```python
from build123d import *

# Parameters (mm, degrees)
SKETCH_1_W          = 87
SKETCH_1_H          = 63
SKETCH_1_W_2        = 83
SKETCH_1_H_2        = 59
EXTRUDE_1_DEPTH     = 5
SKETCH_2_W          = 87
SKETCH_2_H          = 63
EXTRUDE_2_DEPTH     = 2
SKETCH_3_W          = 2.764626384
SKETCH_3_H          = 4.6515936
CUT_EXTRUDE_1_DEPTH = 2
FILLET_1_R          = 2
SKETCH_4_W          = 27.388964673
SKETCH_4_H          = 3.905856672
SKETCH_4_W_2        = 13.70635998
SKETCH_4_H_2        = 4.505719406
SKETCH_4_W_3        = 11.157018238
SKETCH_4_H_3        = 2.851387493
SKETCH_4_W_4        = 3.109085913
SKETCH_4_H_4        = 44.489819457
EXTRUDE_3_DEPTH     = 3.3
SKETCH_5_R          = 2.75
CUT_EXTRUDE_2_DEPTH = 10


with BuildPart() as part:
    # 草图1 → 凸台-拉伸1 (new body)
    with BuildSketch(Plane(origin=(0, 0, 0), x_dir=(0, 0, -1), z_dir=(1, 0, 0))):
        with Locations((3.90387463, 17.013155975)):
            Rectangle(SKETCH_1_W, SKETCH_1_H)
        with Locations((3.90387463, 17.013155975)):
            Rectangle(SKETCH_1_W_2, SKETCH_1_H_2, mode=Mode.SUBTRACT)
    extrude(amount=EXTRUDE_1_DEPTH)

    # 草图2 → 凸台-拉伸2 (add)
    with BuildSketch(Plane(origin=(5, 0, 0), x_dir=(0, 0, -1), z_dir=(1, 0, 0))):
        with Locations((3.90387463, 17.013155975)):
            Rectangle(SKETCH_2_W, SKETCH_2_H)
    extrude(amount=EXTRUDE_2_DEPTH)

    # 草图3 → 切除-拉伸1 (cut)
    with BuildSketch(Plane(origin=(0, 0, -47.40387463), x_dir=(-1, 0, 0), z_dir=(0, 0, -1))):
        with Locations((-3.662779601, -6.806448474)):
            Rectangle(SKETCH_3_W, SKETCH_3_H)
    extrude(amount=-CUT_EXTRUDE_1_DEPTH, mode=Mode.SUBTRACT)

    # 圆角1
    # the kernel refuses this fillet: 2 mm, written as the material it takes off along each edge
    with BuildSketch(Plane(origin=(5, 46.513155975, -45.40387463), x_dir=(1, 0, 0), z_dir=(0, 1, 0))) as fillet_1_piece_1_section:
        Polygon((0, 0), (FILLET_1_R, 0), (FILLET_1_R, FILLET_1_R), (0, FILLET_1_R), align=None)
    fillet_1_piece_1 = extrude(amount=FILLET_1_R, mode=Mode.PRIVATE)
    fillet_1_piece_1 = fillet_1_piece_1 - Plane(origin=(5, 46.513155975, -45.40387463), x_dir=(-0.7071067811865475, 0, 0.7071067811865475), z_dir=(0, 1, 0)) * Sphere(FILLET_1_R, mode=Mode.PRIVATE)
    add(fillet_1_piece_1, mode=Mode.SUBTRACT)
    with BuildSketch(Plane(origin=(5, -12.486844025, -45.40387463), x_dir=(0, 0, -1), z_dir=(1, 0, 0))) as fillet_1_piece_2_section:
        Polygon((0, 0), (FILLET_1_R, 0), (FILLET_1_R, -FILLET_1_R), (0, -FILLET_1_R), align=None)
    fillet_1_piece_2 = extrude(amount=FILLET_1_R, mode=Mode.PRIVATE)
    fillet_1_piece_2 = fillet_1_piece_2 - Plane(origin=(5, -12.486844025, -45.40387463), x_dir=(0, 0.7071067811865474, 0.7071067811865476), z_dir=(1, 0, 0)) * Sphere(FILLET_1_R, mode=Mode.PRIVATE)
    add(fillet_1_piece_2, mode=Mode.SUBTRACT)
    with BuildSketch(Plane(origin=(5, -12.486844025, 37.59612537), x_dir=(1, 0, 0), z_dir=(0, 0, 1))) as fillet_1_piece_3_section:
        Polygon((0, 0), (FILLET_1_R, 0), (FILLET_1_R, -FILLET_1_R), (0, -FILLET_1_R), align=None)
    fillet_1_piece_3 = extrude(amount=FILLET_1_R, mode=Mode.PRIVATE)
    fillet_1_piece_3 = fillet_1_piece_3 - Plane(origin=(5, -12.486844025, 37.59612537), x_dir=(-0.7071067811865475, 0.7071067811865475, 0), z_dir=(0, 0, 1)) * Sphere(FILLET_1_R, mode=Mode.PRIVATE)
    add(fillet_1_piece_3, mode=Mode.SUBTRACT)
    with BuildSketch(Plane(origin=(5, 46.513155975, 37.59612537), x_dir=(0, 0, 1), z_dir=(0, 1, 0))) as fillet_1_piece_4_section:
        Polygon((0, 0), (FILLET_1_R, 0), (FILLET_1_R, FILLET_1_R), (0, FILLET_1_R), align=None)
    fillet_1_piece_4 = extrude(amount=FILLET_1_R, mode=Mode.PRIVATE)
    fillet_1_piece_4 = fillet_1_piece_4 - Plane(origin=(5, 46.513155975, 37.59612537), x_dir=(-0.7071067811865475, 0, -0.7071067811865475), z_dir=(0, 1, 0)) * Sphere(FILLET_1_R, mode=Mode.PRIVATE)
    add(fillet_1_piece_4, mode=Mode.SUBTRACT)
    with BuildSketch(Plane(origin=(5, 48.513155975, -47.40387463), x_dir=(0, 0, 1), z_dir=(-1, 0, 0)), Plane(origin=(5, -14.486844025, -47.40387463), x_dir=(0, 1, 0), z_dir=(-1, 0, 0)), Plane(origin=(-5, -14.486844025, 39.59612537), x_dir=(0, 1, 0), z_dir=(1, 0, 0)), Plane(origin=(-5, 48.513155975, 39.59612537), x_dir=(0, 0, -1), z_dir=(1, 0, 0))) as fillet_1_piece_5:
        with BuildLine():
            CenterArc((FILLET_1_R, -FILLET_1_R), FILLET_1_R, 90, 90)
            Line((0, -FILLET_1_R), (0, 0))
            Line((0, 0), (FILLET_1_R, 0))
        make_face()
    extrude(amount=10, mode=Mode.SUBTRACT)
    with BuildSketch(Plane(origin=(7, 48.513155975, 37.59612537), x_dir=(-1, 0, 0), z_dir=(0, 0, -1))) as fillet_1_piece_6:
        with BuildLine():
            CenterArc((FILLET_1_R, -FILLET_1_R), FILLET_1_R, 90, 90)
            Line((0, -FILLET_1_R), (0, 0))
            Line((0, 0), (FILLET_1_R, 0))
        make_face()
    extrude(amount=83, mode=Mode.SUBTRACT)
    with BuildSketch(Plane(origin=(7, 46.513155975, -47.40387463), x_dir=(0, 0, 1), z_dir=(0, -1, 0))) as fillet_1_piece_7:
        with BuildLine():
            CenterArc((FILLET_1_R, FILLET_1_R), FILLET_1_R, 180, 90)
            Line((0, FILLET_1_R), (0, 0))
            Line((0, 0), (FILLET_1_R, 0))
        make_face()
    extrude(amount=59, mode=Mode.SUBTRACT)
    with BuildSketch(Plane(origin=(7, -14.486844025, -45.40387463), x_dir=(0, 1, 0), z_dir=(0, 0, 1))) as fillet_1_piece_8:
        with BuildLine():
            CenterArc((FILLET_1_R, FILLET_1_R), FILLET_1_R, 180, 90)
            Line((0, FILLET_1_R), (0, 0))
            Line((0, 0), (FILLET_1_R, 0))
        make_face()
    extrude(amount=83, mode=Mode.SUBTRACT)
    with BuildSketch(Plane(origin=(7, -12.486844025, 39.59612537), x_dir=(-1, 0, 0), z_dir=(0, 1, 0))) as fillet_1_piece_9:
        with BuildLine():
            CenterArc((FILLET_1_R, -FILLET_1_R), FILLET_1_R, 90, 90)
            Line((0, -FILLET_1_R), (0, 0))
            Line((0, 0), (FILLET_1_R, 0))
        make_face()
    extrude(amount=59, mode=Mode.SUBTRACT)

    # 草图4 → 凸台-拉伸3 (add)
    with BuildSketch(Plane.ZY.offset(-5)):
        with Locations((13.694482337, -10.533915689)):
            Rectangle(SKETCH_4_W, SKETCH_4_H)
        with Locations((-38.55069464, 44.260296272)):
            Rectangle(SKETCH_4_W_2, SKETCH_4_H_2)
        with Locations((32.017616251, 45.087462229)):
            Rectangle(SKETCH_4_W_3, SKETCH_4_H_3)
        with Locations((36.041582414, 16.563258925)):
            Rectangle(SKETCH_4_W_4, SKETCH_4_H_4)
    extrude(amount=EXTRUDE_3_DEPTH)

    # 草图5 → 切除-拉伸2 (cut)
    with BuildSketch(Plane.ZY.offset(-5)):
        with Locations((-34.13110136, 33.698944985)):
            Circle(SKETCH_5_R)
        with Locations((26.3233521, 33.698944985)):
            Circle(SKETCH_5_R)
        with Locations((-34.13110136, 0.327366965)):
            Circle(SKETCH_5_R)
        with Locations((26.3233521, 0.327366965)):
            Circle(SKETCH_5_R)
    extrude(amount=-CUT_EXTRUDE_2_DEPTH, mode=Mode.SUBTRACT)


solid = part.part
```
Could you check a few things on this model? Use its own coordinates, in mm. A direction names the side the tool comes from. Give positions to 0.01 mm unless a question says otherwise; leave off trailing zeros. Loops run counter-clockwise (first coordinate to the right, second up) from the corner with the lowest first, then second, coordinate; pieces in that order, holes last. Notation, with made-up numbers: (27.5, 79) -> (32.5, 79) arc R13 cw to (32.5, 100) -> close; hole circle Ø4 at (77.5, 88.5). An arc over 180 degrees is marked (long way). Put each result on its own line as item: value.
(1) Imagine slicing it at B-B on z = -40.5. Write out the boundary of the cut face in (x, y), plus the area to 3 significant figures.
Computed:
outline: (0, -14.49) -> (5, -14.49) arc R2 ccw to (7, -12.49) -> (7, 46.51) arc R2 ccw to (5, 48.51) -> (0, 48.51) -> (0, 46.51) -> (1.7, 46.51) -> (1.7, 42.01) -> (5, 42.01) -> (5, -12.49) -> (0, -12.49) -> close
area: 159 mm^2
(2) Imagine slicing it at A-A on x = 4. Write out the boundary of the cut face in (y, z).
Computed:
outline: (-14.49, -45.4) arc R2 ccw to (-12.49, -47.4) -> (-9.13, -47.4) -> (-9.13, -45.4) -> (-12.49, -45.4) -> (-12.49, 0) -> (-8.58, 0) -> (-8.58, 27.39) -> (-12.49, 27.39) -> (-12.49, 37.6) -> (-5.68, 37.6) -> (-5.68, 34.49) -> (38.81, 34.49) -> (38.81, 37.6) -> (43.66, 37.6) -> (43.66, 26.44) -> (46.51, 26.44) -> (46.51, -31.7) -> (42.01, -31.7) -> (42.01, -45.4) -> (-4.48, -45.4) -> (-4.48, -47.4) -> (46.51, -47.4) arc R2 ccw to (48.51, -45.4) -> (48.51, 37.6) arc R2 ccw to (46.51, 39.6) -> (-12.49, 39.6) arc R2 ccw to (-14.49, 37.6) -> close
(3) Thinking about a two-plate mould opening in Y: for faces 1 (the face through (6.399, 16.6, 39.026)), 2 (the face through (2.535, 47.943, -46.802)), 3 (the face through (3, -8.581, 14)), 4 (the face through (4, -9.132, -46)), which applies, pulls with the +Y half, pulls with the -Y half, needs draft (parallel to the pull), parting line crosses it, or undercut?
Computed:
face 1: needs draft
face 2: pulls with the +Y half
face 3: undercut
face 4: undercut
(4) Imagine slicing it at C-C on y = 45.5. Write out the boundary of the cut face in (x, z), plus the area to 3 significant figures.
Computed:
outline: (0, -47.4) -> (5, -47.4) arc R2 ccw to (7, -45.4) -> (7, 37.6) arc R2 ccw to (5, 39.6) -> (0, 39.6) -> (0, 37.6) -> (1.7, 37.6) -> (1.7, 26.44) -> (5, 26.44) -> (5, -31.7) -> (1.7, -31.7) -> (1.7, -45.4) -> (0, -45.4) -> close
area: 274 mm^2
(5) Imagine slicing it at D-D on z = -4.5. Write out the boundary of the cut face in (x, y), plus the area to 3 significant figures.
Computed:
outline: (0, -14.49) -> (5, -14.49) arc R2 ccw to (7, -12.49) -> (7, 46.51) arc R2 ccw to (5, 48.51) -> (0, 48.51) -> (0, 46.51) -> (5, 46.51) -> (5, -12.49) -> (0, -12.49) -> close
area: 144 mm^2
(6) Please list where these lines run through material, in increasing order: probe 1 along Z at (x, y) = (4.75, 12); probe 2 along Z at (x, y) = (1.5, 3); probe 3 along Y at (x, z) = (1, 25). Write a range as [from, to].
Computed:
probe 1: [-47.4, -45.4], [34.49, 39.6]
probe 2: [-47.4, -45.4], [37.6, 39.6]
probe 3: [-14.49, -12.49], [46.51, 48.51]
(7) For faces 5 (the face through (4, -4.481, -46)), 6 (the face through (2, 48.513, -3)), 7 (the face through (3, 16, 34.487)), which set-ups out of +Z, -Z, +X, -X, +Y, -Y let a thin tool reach every point of the face, with its end or its side?
Computed:
face 5: -Z
face 6: +Z, -Z, +X, -X, +Y
face 7: -X
(8) I'm going to push flat-ended pins straight in: pin 1 Ø3.5 at (y, z) = (44, -42) entering from -X; pin 2 Ø0.6 at (y, z) = (-6, -46.5) entering from +X; pin 3 Ø6 at (y, z) = (7, -35) entering from -X. Where does each tip first touch, or does it pass through?
Computed:
pin 1: x = 1.7
pin 2: x = 6.83
pin 3: x = 5
